Here's how the part is built. I have some questions about the finished solid (model axes, mm). Face numbers are marked on the shaded views. A direction names the side the tool comes from. Round coordinates to 2 decimals unless told otherwise and drop trailing zeros. Write each loop counter-clockwise with the first axis right and the second up, starting at its lowest first coordinate (ties: lowest second). Pieces come first, ordered by that corner, then holes. Notation, with made-up numbers: (-28.75, 89.25) - (9.25, 89.25) arc R12 cw to (9.25, 100.25) - close; hole circle Ø5 at (-31, 19). An arc over 180 degrees is marked (long way). One line per item, written item: value. Start each with the question number.
Item 1: If I drill on line 1 (Y direction, x = -37.5, z = 6); line 2 (Z direction, x = -1.5, y = 7.75); line 3 (X direction, y = 2.5, z = 5.5), over which ranges is the centre line in solid material (lowest first)?
Item 2: Imagine slicing it at A-A, the plane y = 6.75. Please give me the cut outline in (x, z).
Item 3: For the marked faces 4 and 5, which set-ups out of +Z, -Z, +X, -X, +Y, -Y let a thin tool reach every point of the face, with its end or its side?
Item 4: Imagine slicing it at B-B, the plane z = 8.5. Please give me the cut outline in (x, y).
Item 5: Thinking about a two-plate mould opening in Z: for the marked faces 1, 2 and 3, which applies, released by +Z, released by -Z, zero draft, split by the parting line, or undercut?
Item 6: For P1, Ø6, axis at x = -37.5, y = 0, coming from the -Z side, with a flat end and sliding along its axis, tell me the tip position at first contact or that it passes through.
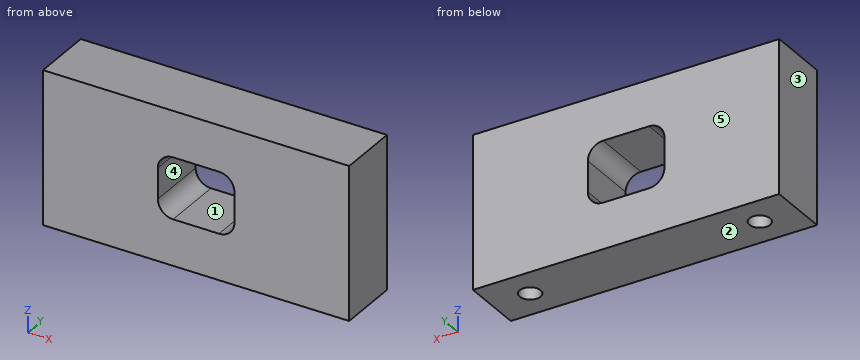
```python
from build123d import *

# Parameters (mm, degrees)
F0_W     = 100
F0_H     = 50
F1_DEPTH = 10
F3_D     = 6.8
F3_DEPTH = 15.75
F3_TIP   = 2.0429261047


with BuildPart() as f1:
    # F0 (on Front) → F1 (new body, symmetric)
    with BuildSketch(Plane.XZ):
        with Locations((0, 25)):
            Rectangle(F0_W, F0_H)
        with BuildLine():
            ThreePointArc((12.5, 20), (11.0355339059, 16.4644660941), (7.5, 15))
            Line((7.5, 15), (-7.5, 15))
            ThreePointArc((-7.5, 15), (-11.0355339059, 16.4644660941), (-12.5, 20))
            Line((-12.5, 20), (-12.5, 30))
            ThreePointArc((-12.5, 30), (-11.0355339059, 33.5355339059), (-7.5, 35))
            Line((-7.5, 35), (7.5, 35))
            ThreePointArc((7.5, 35), (11.0355339059, 33.5355339059), (12.5, 30))
            Line((12.5, 30), (12.5, 20))
        make_face(mode=Mode.SUBTRACT)
    extrude(amount=F1_DEPTH, both=True)

    # F3
    with Locations(Plane(origin=(0, 0, 0), x_dir=(1, 0, 0), z_dir=(0, 0, -1))):
        with Locations((-37.5, 0), (37.5, 0)):
            Hole(F3_D / 2, depth=F3_DEPTH)
            with Locations((0, 0, -(F3_DEPTH + F3_TIP / 2))):  # 118° drill point
                Cone(0, F3_D / 2, F3_TIP, mode=Mode.SUBTRACT)


solid = f1.part
```
Values follow:
1. line 1: y = -10 to -3.4, 3.4 to 10
1. line 2: z = 0 to 15, 35 to 50
1. line 3: x = -50 to -39.8, -35.2 to 35.2, 39.8 to 50
2. outline: (-50, 0) - (50, 0) - (50, 50) - (-50, 50) - close; hole (-12.5, 20) arc R5 ccw to (-7.5, 15) - (7.5, 15) arc R5 ccw to (12.5, 20) - (12.5, 30) arc R5 ccw to (7.5, 35) - (-7.5, 35) arc R5 ccw to (-12.5, 30) - close
3. face 4: +Y, -Y
3. face 5: +Z, -Z, +X, -X, +Y
4. outline: (-50, -10) - (50, -10) - (50, 10) - (-50, 10) - close; hole circle Ø6.8 at (-37.5, 0); hole circle Ø6.8 at (37.5, 0)
5. face 1: undercut
5. face 2: released by -Z
5. face 3: zero draft
6. P1: stops at z = 15.99
